For this review, take the finished solid that the model builds, in its own axes (mm). A direction names the side the tool comes from. Round coordinates to 2 decimals unless told otherwise and drop trailing zeros. Write each loop counter-clockwise with the first axis right and the second up, starting at its lowest first coordinate (ties: lowest second). Pieces come first, ordered by that corner, then holes.
from build123d import *

# Parameters (mm, degrees)
SKETCH1_W           = 279.4
SKETCH1_H           = 30.48
BOSS_EXTRUDE1_DEPTH = 9.525
SKETCH2_W           = 12.7
SKETCH2_H           = 9.525
BOSS_EXTRUDE2_DEPTH = 9.525
SKETCH4_W           = 76.2
SKETCH4_H           = 30.48
SKETCH4_W_2         = 50.8
CUT_EXTRUDE1_DEPTH  = 4.7625


with BuildPart() as part:
    # Sketch1 → Boss-Extrude1 (new body)
    with BuildSketch(Plane(origin=(0, 0, 0), x_dir=(1, 0, 0), z_dir=(0, 1, 0))):
        Rectangle(SKETCH1_W, SKETCH1_H)
    extrude(amount=BOSS_EXTRUDE1_DEPTH)

    # Sketch2 → Boss-Extrude2 (add)
    with BuildSketch(Plane(origin=(139.7, 0, 0), x_dir=(0, 0, -1), z_dir=(1, 0, 0))):
        with Locations((0, 4.7625)):
            Rectangle(SKETCH2_W, SKETCH2_H)
    boss_extrude2 = extrude(amount=BOSS_EXTRUDE2_DEPTH)

    # Mirror1: Boss-Extrude2 across plane
    add(boss_extrude2.mirror(Plane(origin=(0, 0, 0), x_dir=(0, 0, 1), z_dir=(1, 0, 0))))

    # Sketch4 → Cut-Extrude1 (cut)
    with BuildSketch(Plane(origin=(0, 9.525, 0), x_dir=(1, 0, 0), z_dir=(0, 1, 0))):
        Rectangle(SKETCH4_W, SKETCH4_H)
        with Locations((88.9, 0)):
            Rectangle(SKETCH4_W_2, SKETCH4_H)
        with Locations((-88.9, 0)):
            Rectangle(SKETCH4_W_2, SKETCH4_H)
    extrude(amount=-CUT_EXTRUDE1_DEPTH, mode=Mode.SUBTRACT)


solid = part.part
(1) We need section C-C, the plane x = 5.5. Give the boundary of the cut face in (y, z).
Geometry check:
outline: (0, -15.24) - (4.76, -15.24) - (4.76, 15.24) - (0, 15.24) - close
(2) For pin 1 Ø9 at (x, z) = (-101.5, 7) entering from +Y; pin 2 Ø3 at (x, y) = (143.5, 6.5) entering from +Z; pin 3 Ø2.5 at (y, z) = (4, 11.5) entering from +X; pin 4 Ø2 at (x, z) = (-34, 10) entering from -Y, all flat-tipped, find the tip position at first contact; note any pin that passes through.
Geometry check:
pin 1: stops at y = 4.76
pin 2: stops at z = 6.35
pin 3: stops at x = 139.7
pin 4: stops at y = 0
(3) We need section B-B, the plane z = -3.5. Give the boundary of the cut face in (x, y) (1 decimal).
Geometry check:
outline: (-149.2, 0) - (149.2, 0) - (149.2, 9.5) - (114.3, 9.5) - (114.3, 4.8) - (63.5, 4.8) - (63.5, 9.5) - (38.1, 9.5) - (38.1, 4.8) - (-38.1, 4.8) - (-38.1, 9.5) - (-63.5, 9.5) - (-63.5, 4.8) - (-114.3, 4.8) - (-114.3, 9.5) - (-149.2, 9.5) - close
(4) Mouldability with a two-part tool opening along X and no side actions: class faces 5 (the face through (-114.3, 7, 0)), 6 (the face through (-139.7, 5, -11)), 7 (the face through (51, 9.525, 0)) as pulls with the +X half, pulls with the -X half, needs draft (parallel to the pull), parting line crosses it, or undercut.
Geometry check:
face 5: undercut
face 6: pulls with the -X half
face 7: needs draft
(5) We need section A-A, the plane y = 6.5. Give the boundary of the cut face in (x, z) (3 decimals).
Geometry check:
outline: (-149.225, -6.35) - (-139.7, -6.35) - (-139.7, -15.24) - (-114.3, -15.24) - (-114.3, 15.24) - (-139.7, 15.24) - (-139.7, 6.35) - (-149.225, 6.35) - close; (-63.5, -15.24) - (-38.1, -15.24) - (-38.1, 15.24) - (-63.5, 15.24) - close; (38.1, -15.24) - (63.5, -15.24) - (63.5, 15.24) - (38.1, 15.24) - close; (114.3, -15.24) - (139.7, -15.24) - (139.7, -6.35) - (149.225, -6.35) - (149.225, 6.35) - (139.7, 6.35) - (139.7, 15.24) - (114.3, 15.24) - close
(6) For line 1 along X through (y, z) = (8.5, -7); line 2 along X through (y, z) = (7.75, 0.5) (3 decimals); line 3 along X through (y, z) = (2.75, -11), list the stretches that pass through material, from the lowest coordinate up.
Geometry check:
line 1: x = -139.7 to -114.3, -63.5 to -38.1, 38.1 to 63.5, 114.3 to 139.7
line 2: x = -149.225 to -114.3, -63.5 to -38.1, 38.1 to 63.5, 114.3 to 149.225
line 3: x = -139.7 to 139.7
(7) For faces 1 (the face through (-144, 5, -6.35)), 2 (the face through (139.7, 5, -11)), 3 (the face through (-38.1, 7, 0)), 4 (the face through (139.7, 5, 11)), list the 3-axis set-ups (+Z, -Z, +X, -X, +Y, -Y) from which the entire face can be reached by the end or side of a thin tool; tool diameter is ignored.
Geometry check:
face 1: -Z, -X, +Y, -Y
face 2: -Z, +X, +Y, -Y
face 3: +Z, -Z, +Y
face 4: +Z, +X, +Y, -Y
